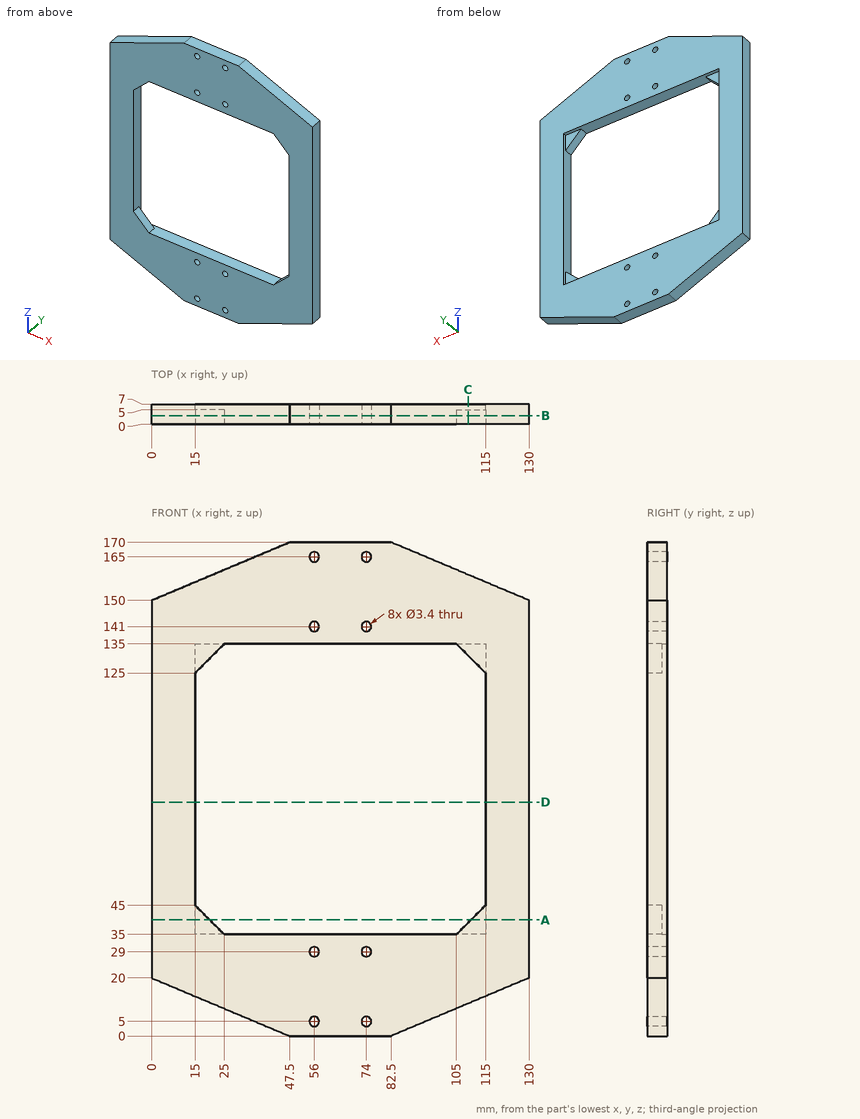
Source: three-view drawing plus pictorial views. Frame: mm from the lowest corner of the part. Round coordinates to 2 decimals unless told otherwise and drop trailing zeros. Loops run counter-clockwise (first coordinate to the right, second up) from the corner with the lowest first, then second, coordinate; pieces in that order, holes last.
Q1. Section C-C on x = 109. Return loops of the section in (y, z).
Q2. Section B-B on y = 3. State how many separate pieces and enclosed holes the cut face has, plus the area to 3 significant figures.
Q3. Section D-D on z = 80.5. Return loops of the section in (x, y), plus the area to 3 significant figures.
Q4. Section A-A on z = 40. Return loops of the section in (x, y).
Q5. Pin query (flat end, axial travel): P1, Ø2, axis at x = 74, z = 141, coming from the -Y side; P2, Ø3, axis at x = 18.5, z = 127.5, coming from the +Y side; P3, Ø1.5, axis at x = 114, y = 2, coming from the +Z side. Return the tip coordinate at first contact, or that it passes through.
Q6. Material intervals for L1, parallel to X at y = 4.25, z = 5 (3 decimals); L2, parallel to X at y = 6.5, z = 60; L3, parallel to Z at x = 59.5, y = 4, sorted ascending.
Evaluation:
1. outline: (0, 11.16) - (7, 11.16) - (7, 35) - (5, 35) - (5, 39) - (0, 39) - close; (0, 131) - (5, 131) - (5, 135) - (7, 135) - (7, 158.84) - (0, 158.84) - close
2. separate pieces: 1
2. enclosed holes: 9
2. area: 10,300 mm2
3. outline: (0, 0) - (15, 0) - (15, 7) - (0, 7) - close; (115, 0) - (130, 0) - (130, 7) - (115, 7) - close
3. area: 210 mm2
4. outline: (0, 0) - (20, 0) - (20, 5) - (15, 5) - (15, 7) - (0, 7) - close; (110, 0) - (130, 0) - (130, 7) - (115, 7) - (115, 5) - (110, 5) - close
5. P1: passes through
5. P2: stops at y = 5
5. P3: stops at z = 157.05
6. L1: x = 35.625 to 54.3, 57.7 to 72.3, 75.7 to 94.375
6. L2: x = 0 to 15, 115 to 130
6. L3: z = 0 to 35, 135 to 170
